```python
from build123d import *

# Parameters (mm, degrees)
F0_W          = 76.2
F0_H          = 76.2
F1_DEPTH      = 3.175
F1_DEPTH_BACK = 3.175
F2_R          = 11.1125
F3_DEPTH      = 25.4
F5_DEPTH      = 25.4
F7_DEPTH      = 25.4
F9_DEPTH      = 25.4
F10_DEPTH     = 25.4


with BuildPart() as f1:
    # F0 (on Top) → F1 (new body, two sides)
    with BuildSketch(Plane.XY) as f1_sk:
        Rectangle(F0_W, F0_H)
    extrude(amount=F1_DEPTH)
    extrude(f1_sk.sketch, amount=-F1_DEPTH_BACK)

    # F2 (on face) → F3 (cut)
    with BuildSketch(Plane.XY.offset(3.175)):
        Circle(F2_R)
    extrude(amount=-F3_DEPTH, mode=Mode.SUBTRACT)

    # F4 (on face) → F5 (cut)
    with BuildSketch(Plane.XY.offset(3.175)):
        with BuildLine():
            ThreePointArc((-1.1282384551, 15.834857214), (0, 15.875), (1.1282384551, 15.834857214))
            ThreePointArc((1.1282384551, 15.834857214), (19.6798871657, 16.6861460125), (38.1, 19.05))
            Line((38.1, 19.05), (38.1, 38.1))
            Line((38.1, 38.1), (-38.1, 38.1))
            Line((-38.1, 38.1), (-38.1, 19.05))
            ThreePointArc((-38.1, 19.05), (-19.6798871657, 16.6861460125), (-1.1282384551, 15.834857214))
        make_face()
        with BuildLine():
            ThreePointArc((38.1, -19.05), (19.3632933861, -16.6846942182), (0.4955788466, -15.867262732))
            ThreePointArc((0.4955788466, -15.867262732), (0, -15.875), (-0.4955788466, -15.867262732))
            ThreePointArc((-0.4955788466, -15.867262732), (-19.3632933861, -16.6846942182), (-38.1, -19.05))
            Line((-38.1, -19.05), (-38.1, -38.1))
            Line((-38.1, -38.1), (38.1, -38.1))
            Line((38.1, -38.1), (38.1, -19.05))
        make_face()
    extrude(amount=-F5_DEPTH, mode=Mode.SUBTRACT)

    # F6 (on face) → F7 (cut)
    with BuildSketch(Plane.XY.offset(3.175)):
        with BuildLine():
            ThreePointArc((-31.8240671696, -18.0829596142), (-36.2945422432, -10.1630092501), (-38.1, -1.2494755264))
            Line((-38.1, -1.2494755264), (-38.1, -19.05))
            ThreePointArc((-38.1, -19.05), (-34.9653769343, -18.5447820191), (-31.8240671696, -18.0829596142))
        make_face()
        with BuildLine():
            Line((38.1, -19.05), (38.1, -0.7031421254))
            ThreePointArc((38.1, -0.7031421254), (36.375777878, -9.9035605014), (31.8240671696, -18.0829596142))
            ThreePointArc((31.8240671696, -18.0829596142), (34.9653769343, -18.5447820191), (38.1, -19.05))
        make_face()
        with BuildLine():
            Line((38.1, 0.6947725682), (38.1, 19.05))
            ThreePointArc((38.1, 19.05), (34.9662556013, 18.5393499989), (31.8256799416, 18.072550357))
            ThreePointArc((31.8256799416, 18.072550357), (36.3762194276, 9.8939680843), (38.1, 0.6947725682))
        make_face()
        with BuildLine():
            ThreePointArc((-38.1, 1.2410984186), (-36.2949953659, 10.153416681), (-31.8256799416, 18.072550357))
            ThreePointArc((-31.8256799416, 18.072550357), (-34.9662556013, 18.5393499989), (-38.1, 19.05))
            Line((-38.1, 19.05), (-38.1, 1.2410984186))
        make_face()
    extrude(amount=-F7_DEPTH, mode=Mode.SUBTRACT)

    # F8 (on face) → F9 (cut)
    with BuildSketch(Plane.XY.offset(3.175)):
        Polygon((-21.43125, 11.4536878589), (-24.60625, 11.4536878589), (-27.78125, 11.4536878589), (-27.78125, 6.3736878589), (-34.13125, 6.3736878589), (-34.13125, 0.0236878589), (-27.78125, 0.0236878589), (-27.78125, -11.4063121411), (-21.43125, -11.4063121411), (-21.43125, 0.0236878589), (-15.08125, 0.0236878589), (-15.08125, 6.3736878589), (-21.43125, 6.3736878589), align=None)
        Polygon((21.4206709149, -11.47287669), (24.5575709149, -11.47287669), (27.7706709149, -11.47287669), (27.7706709149, -6.39287669), (34.1206709149, -6.39287669), (34.1206709149, -0.04287669), (27.7706709149, -0.04287669), (27.7706709149, 11.38712331), (21.4206709149, 11.38712331), (21.4206709149, -0.04287669), (15.0706709149, -0.04287669), (15.0706709149, -6.39287669), (21.4206709149, -6.39287669), align=None)
    extrude(amount=-F9_DEPTH, mode=Mode.SUBTRACT)

    # F8 (on face) → F10 (cut)
    with BuildSketch(Plane.XY.offset(3.175)):
        Polygon((-21.43125, 11.4536878589), (-24.60625, 11.4536878589), (-27.78125, 11.4536878589), (-27.78125, 6.3736878589), (-34.13125, 6.3736878589), (-34.13125, 0.0236878589), (-27.78125, 0.0236878589), (-27.78125, -11.4063121411), (-21.43125, -11.4063121411), (-21.43125, 0.0236878589), (-15.08125, 0.0236878589), (-15.08125, 6.3736878589), (-21.43125, 6.3736878589), align=None)
        Polygon((21.4206709149, -11.47287669), (24.5575709149, -11.47287669), (27.7706709149, -11.47287669), (27.7706709149, -6.39287669), (34.1206709149, -6.39287669), (34.1206709149, -0.04287669), (27.7706709149, -0.04287669), (27.7706709149, 11.38712331), (21.4206709149, 11.38712331), (21.4206709149, -0.04287669), (15.0706709149, -0.04287669), (15.0706709149, -6.39287669), (21.4206709149, -6.39287669), align=None)
    extrude(amount=-F10_DEPTH, mode=Mode.SUBTRACT)


solid = f1.part
```
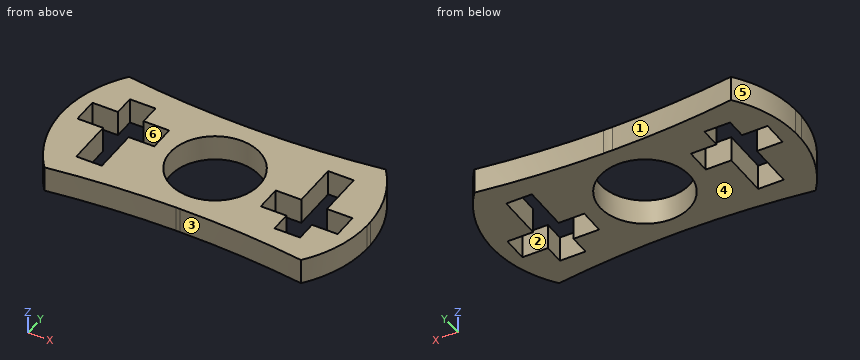
Geometry: final body of the model. Coordinates: model frame, mm. Face numbers are marked on the shaded views. A direction names the side the tool comes from. Coordinates: 2 decimals unless noted, no trailing zeros. Write each loop counter-clockwise with the first axis right and the second up, starting at its lowest first coordinate (ties: lowest second). Pieces come first, ordered by that corner, then holes. Notation, with made-up numbers: M 82.25,82.5 L 116.25,82.5 A21 ccw 116.25,108.5 Z; hole C 64,82 d11. An arc over 180 degrees is marked long. Answer as CSV lines item,"result". Start each with the question number.
Q1. Cut plane A-A on y = -10. Return the cut outline in (x, z) (3 decimals).
Q2. Reachability of the marked faces 1, 2 and 3 from +Z, -Z, +X, -X, +Y, -Y: full face, straight path, thin tool, end or side. Return the list, or none.
Q3. Mould query, pull axis X, two halves, no side actions, for the marked faces 4, 5 and 6. Classes: released by +X, released by -X, zero draft, split by the parting line, or undercut.
Q4. Cut plane C-C on y = 8.5. Return the cut outline in (x, z) (3 decimals), then the cut area to 3 significant figures.
Q5. Cut plane D-D on x = 5. Return the cut outline in (y, z) (3 decimals).
Q6. Cut plane B-B on x = -25.5. Return the cut outline in (y, z) (3 decimals), then the cut area to 3 significant figures.
Q7. Pin query (flat end, axial travel): P1, Ø1.5, axis at x = 2.5, z = -1, coming from the +Y side; P2, Ø1.5, axis at x = 4, z = -0.5, coming from the -Y side; P3, Ø1.9, axis at x = 31, z = -0.5, coming from the -Y side; P4, Ø1.9, axis at x = 17, z = 1.5, coming from the +Y side. Return the tip coordinate at first contact, or that it passes through.
Q8. Line query: line 1 (Y direction, x = 0, z = -0.25) (1 decimal); line 2 (X direction, y = 4.5, z = 1.5); line 3 (X direction, y = -10, z = -0.5). Output: solid intervals per line, ascending. Write a range as from..to.
Findings below:
1,outline,"M -36.355,-3.175 L -27.781,-3.175 L -27.781,3.175 L -36.355,3.175 Z; M -21.431,-3.175 L -4.846,-3.175 L -4.846,3.175 L -21.431,3.175 Z; M 4.846,-3.175 L 21.421,-3.175 L 21.421,3.175 L 4.846,3.175 Z; M 27.771,-3.175 L 36.341,-3.175 L 36.341,3.175 L 27.771,3.175 Z"
2,face 1,"+Z, -Z, +Y"
2,face 2,"+Z, -Z"
2,face 3,"+Z, -Z, -Y"
3,face 4,"zero draft"
3,face 5,"released by -X"
3,face 6,"undercut"
4,outline,"M -36.855,-3.175 L -27.781,-3.175 L -27.781,3.175 L -36.855,3.175 Z; M -21.431,-3.175 L -7.158,-3.175 L -7.158,3.175 L -21.431,3.175 Z; M 7.158,-3.175 L 21.421,-3.175 L 21.421,3.175 L 7.158,3.175 Z; M 27.771,-3.175 L 36.84,-3.175 L 36.84,3.175 L 27.771,3.175 Z"
4,area,"296 mm2"
5,outline,"M -15.921,-3.175 L -9.924,-3.175 L -9.924,3.175 L -15.921,3.175 Z; M 9.924,-3.175 L 15.887,-3.175 L 15.887,3.175 L 9.924,3.175 Z"
6,outline,"M -17.287,-3.175 L -11.406,-3.175 L -11.406,3.175 L -17.287,3.175 Z; M 11.454,-3.175 L 17.268,-3.175 L 17.268,3.175 L 11.454,3.175 Z"
6,area,"74.3 mm2"
7,P1,"stops at y = 15.86"
7,P2,"stops at y = -15.92"
7,P3,"stops at y = -18.08"
7,P4,"stops at y = 16.54"
8,line 1,"y = -15.9..-11.1, 11.1..15.9"
8,line 2,"x = -37.78..-34.13, -15.08..-10.16, 10.16..21.42, 27.77..37.76"
8,line 3,"x = -36.35..-27.78, -21.43..-4.85, 4.85..21.42, 27.77..36.34"
